Autodesk Inventor part; units mm, degrees
ref_plane "YZ Plane" through (0, 0, 0) normal (1, 0, 0) x (0, 1, 0)
ref_plane "XZ Plane" through (0, 0, 0) normal (0, 1, 0) x (-1, 0, 0)
ref_plane "XY Plane" through (0, 0, 0) normal (0, 0, 1) x (1, 0, 0)
sketch "Sketch5" plane through (0, 0, 0) normal (0, 0, 1) x (1, 0, 0)
  line L0 (0, 0) -> (50, 0)
  line L1 (50, 0) -> (50, 20)
  line L2 (50, 20) -> (0, 20)
  line L3 (0, 20) -> (0, 0)
  circle A0 centre (10, 10) radius 3
  circle A1 centre (40, 10) radius 3
  dimension "d43" = 50
  dimension "d44" = 20
  dimension "d47" = 6
  dimension "d48" = 6
  dimension "d49" = 10
  dimension "d50" = 10
  dimension "d51" = 10
  dimension "d52" = 10
extrude "Extrusion5" add sketch "Sketch5" along normal blind 5
sketch "Sketch8" plane through (0, 20, 0) normal (0, 1, 0) x (1, 0, 0)
  line L0 (50, 0) -> (0, 0)
  line L1 (0, 0) -> (0, -5)
  line L2 (50, -5) -> (0, -5)
  line L3 (50, 0) -> (50, -5)
  line L4 (0, -5) -> (50, -5)
  line L5 (50, -5) -> (50, 30)
  line L6 (50, 30) -> (0, 30)
  line L7 (0, 30) -> (0, -5)
  line L8 (0, 30) -> (0, 15) construction
  line L9 (0, 0) -> (0, 25) construction
  dimension "d55" = 50
  dimension "d56" = 35
extrude "Extrusion6" add sketch "Sketch8" against normal blind 3 contours L0 L7 L6 L5
sketch "Sketch10" plane through (0, 17, 0) normal (0, -1, 0) x (1, 0, 0)
  line L0 (0, 0) -> (50, 0)
  line L1 (50, -30) -> (50, 0)
  line L2 (25, 0) -> (25, -50.2425) construction
  line L3 (25, 0) -> (25, -20) construction
  line L4 (25, -20) -> (44.8883, -20) construction
  line L5 (44.8883, -20) -> (4.4649, -20) construction
  circle A0 centre (25, -20) radius 5
  circle A1 centre (25, -20) radius 7
  dimension "d68" = 20
  dimension "d69" = 10
  dimension "d70" = 14
extrude "Extrusion8" add sketch "Sketch10" along normal blind 5
properties part number "z smooth rod mount" material "ABS Plastic"
The listing builds one solid part. Answer for the finished solid, in the listing's coordinates (mm). A direction names the side the tool comes from. Coordinates: 2 decimals unless noted, no trailing zeros. Write each loop counter-clockwise with the first axis right and the second up, starting at its lowest first coordinate (ties: lowest second). Pieces come first, ordered by that corner, then holes. Notation, with made-up numbers: (56, -5) - (60, -5) arc R17 ccw to (60, 6) - close; hole circle Ø5 at (31, 82.5). An arc over 180 degrees is marked (long way). Return JSON: item names as keys, results as strings. Group by question number.
Q1. Which of the six approach directions +Z, -Z, +X, -X, +Y, -Y give full straight-line access (tool end or side, diameter ignored) to faces 1 (the flat face through (23, 12, -15)), 2 (the flat face through (25, 17, -12)), 3 (the flat face through (50, 17.4, -6.1))?
Q2. For a pull along Y with two mould halves and no side action, classify faces 4 (the flat face through (25, 20, -13)), 5 (the cylindrical face through (11.61, 7.47, 2.46)), 6 (the flat face through (25, 0, 2)) as +Y half, -Y half, draft (parallel to the pull), parting line (faces both ways), or undercut.
Q3. The part is cut by section A-A on x = 40. Write down the section's boundary in (y, z), and give its area (3 significant figures).
Q4. Find the intervals of material crossed by line 1 along Y through (x, z) = (10, 3.45); line 2 along Z through (x, y) = (21, 11); line 3 along Y through (x, z) = (11, -4), in increasing order. Write a range as [from, to].
Q5. The part is cut by section C-C on z = -20. Write down the section's boundary in (x, y), and give its area (3 significant figures).
Q6. Flat-ended cylindrical pins translate along their axes: pin 1 Ø15 at (x, z) = (34.5, -18.5) entering from -Y; pin 2 Ø9 at (x, z) = (25, -20) entering from -Y; pin 3 Ø8 at (y, z) = (7, -20.5) entering from +X; pin 4 Ø9.5 at (x, y) = (10, 10) entering from -Z. Find the tip coordinate at first contact, or state that the pin passes through.
Q7. The part is cut by section D-D on x = 25. Write down the section's boundary in (y, z).
Q8. The part is cut by section B-B on y = 10. Write down the section's boundary in (x, z).
Evaluation:
{
 "1": {"face 1": "-Z, +X, -X, -Y", "face 2": "-Y", "face 3": "+Z, -Z, +X, +Y, -Y"},
 "2": {"face 4": "+Y half", "face 5": "undercut", "face 6": "-Y half"},
 "3": {"outline": "(0, 0) - (7, 0) - (7, 5) - (0, 5) - close; (13, 0) - (17, 0) - (17, -30) - (20, -30) - (20, 5) - (13, 5) - close", "area": "160 mm2"},
 "4": {"line 1": "y = [0, 7], [13, 20]", "line 2": "z = [0, 5]", "line 3": "y = [17, 20]"},
 "5": {"outline": "(0, 17) - (18, 17) - (18, 12) - (20, 12) - (20, 17) - (30, 17) - (30, 12) - (32, 12) - (32, 17) - (50, 17) - (50, 20) - (0, 20) - close", "area": "170 mm2"},
 "6": {"pin 1": "stops at y = 12", "pin 2": "stops at y = 17", "pin 3": "passes through", "pin 4": "stops at z = 0"},
 "7": {"outline": "(0, 0) - (17, 0) - (17, -13) - (12, -13) - (12, -15) - (17, -15) - (17, -25) - (12, -25) - (12, -27) - (17, -27) - (17, -30) - (20, -30) - (20, 5) - (0, 5) - close"},
 "8": {"outline": "(0, 0) - (7, 0) - (7, 5) - (0, 5) - close; (13, 0) - (37, 0) - (37, 5) - (13, 5) - close; (43, 0) - (50, 0) - (50, 5) - (43, 5) - close"}
}
